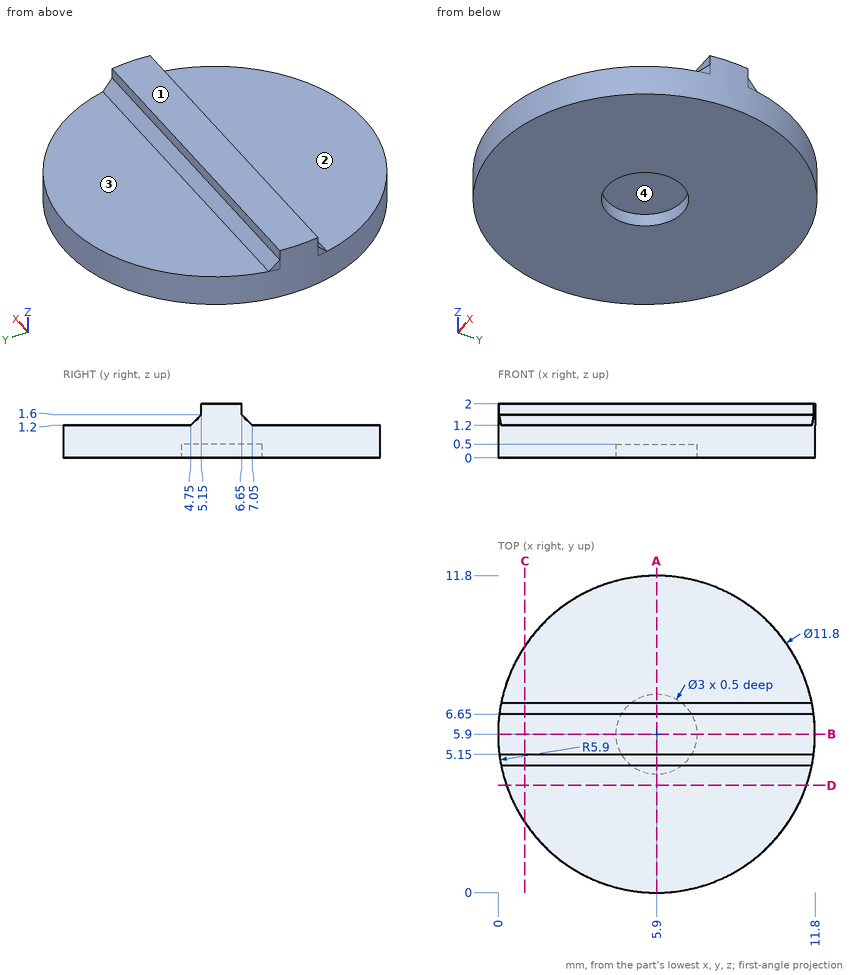
Geometry check sheet. Reference: drawing and pictorial views, mm from the part's lowest x, y, z. A direction names the side the tool comes from. Round coordinates to 2 decimals unless told otherwise and drop trailing zeros. Loops run counter-clockwise (first coordinate to the right, second up) from the corner with the lowest first, then second, coordinate; pieces in that order, holes last. Notation, with made-up numbers: M -4.5,13.5 L 22.5,13.5 A14 ccw 22.5,28.5 Z; hole C -0.75,13.25 d2. An arc over 180 degrees is marked long. Return JSON: item names as keys, results as strings. Group by question number.
(1) Go/stop test with flat-tipped pins: pin 1 (1.4 mm diameter, centred on x = 6, y = 2.5, fed in from +Z); pin 2 (0.9 mm diameter, centred on x = 5, y = 6, fed in from -Z). Record where each tip stops, or that it passes through.
(2) Section check C-C, the plane x = 1. Enter the section's corners in (y, z).
(3) Scan lines: line 1 along Y through (x, z) = (5.9, 0.2); line 2 along Z through (x, y) = (2.75, 2.5); line 3 along Y through (x, z) = (8.75, 0.25). Record each from-to range of solid material in increasing order. Write a range as [from, to].
(4) Mould release check, pull along X, two halves, no side actions. Record for the marked faces 3 and 4: pulls with the +X half, pulls with the -X half, needs draft (parallel to the pull), parting line crosses it, or undercut.
(5) Section check B-B, the plane y = 5.9. Enter the section's corners in (x, z).
(6) Section check D-D, the plane y = 4. Enter the section's corners in (x, z).
(7) Section check A-A, the plane x = 5.9. Enter the section's corners in (y, z), and give its area (3 significant figures).
(8) Set-up check for the marked faces 1 and 2: record each of +Z, -Z, +X, -X, +Y, -Y from which the full face is reachable in a straight line by a thin tool's end or side.
Data:
{
 "1": {"pin 1": "z = 1.2", "pin 2": "z = 0.5"},
 "2": {"outline": "M 2.61,0 L 9.19,0 L 9.19,1.2 L 7.05,1.2 L 6.65,1.6 L 6.65,2 L 5.15,2 L 5.15,1.6 L 4.75,1.2 L 2.61,1.2 Z"},
 "3": {"line 1": "[0, 4.4], [7.4, 11.8]", "line 2": "[0, 1.2]", "line 3": "[0.73, 11.07]"},
 "4": {"face 3": "needs draft", "face 4": "undercut"},
 "5": {"outline": "M 0,0 L 4.4,0 L 4.4,0.5 L 7.4,0.5 L 7.4,0 L 11.8,0 L 11.8,2 L 0,2 Z"},
 "6": {"outline": "M 0.31,0 L 11.49,0 L 11.49,1.2 L 0.31,1.2 Z"},
 "7": {"outline": "M 0,0 L 4.4,0 L 4.4,0.5 L 7.4,0.5 L 7.4,0 L 11.8,0 L 11.8,1.2 L 7.05,1.2 L 6.65,1.6 L 6.65,2 L 5.15,2 L 5.15,1.6 L 4.75,1.2 L 0,1.2 Z", "area": "14.0 mm²"},
 "8": {"face 1": "+Z, +X, -X, +Y, -Y", "face 2": "+Z, +X, -X, -Y"}
}
